Work out the finished part from the listing and answer in its coordinate system (mm). Face numbers are marked on the shaded views. Round coordinates to 2 decimals unless told otherwise and drop trailing zeros. Write each loop counter-clockwise with the first axis right and the second up, starting at its lowest first coordinate (ties: lowest second). Pieces come first, ordered by that corner, then holes.
1. Flat-ended cylindrical pins translate along their axes: pin 1 Ø7 at (x, y) = (-130, 0) entering from -Z; pin 2 Ø4 at (x, z) = (-96.5, 11.5) entering from -Y; pin 3 Ø1 at (y, z) = (64, 7) entering from -X. Find the tip coordinate at first contact, or state that the pin passes through.
2. Find section C-C (y = 0). Write down the section's boundary in (x, z).
3. Find section A-A (z = 12.5). Write down the section's boundary in (x, y).
4. Determine the mould class of the marked faces 1, 2 and 3 for opening direction Y: pulls with the +Y half, pulls with the -Y half, needs draft (parallel to the pull), parting line crosses it, or undercut.
5. Find section B-B (x = -130). Write down the section's boundary in (y, z).
6. Straight lines are drawn through the part: probe 1 along Y at (x, z) = (-130, 9.5); probe 2 along X at (y, z) = (0, 12.25); probe 3 along Z at (x, y) = (-130.5, -5). For each, find the intervals that lie inside material, in ascending order.
7. Find section D-D (y = 98). Write down the section's boundary in (x, z), and give its area (3 significant figures).
```python
from build123d import *

# Parameters (mm, degrees)
ESQUISSE2_R             = 2.75
BOSS_EXTRU_1_DEPTH      = 15
ENL_V_MAT_EXTRU_1_DEPTH = 36
CONG_1_R                = 30
CONG_2_R                = 30
CONG_3_R                = 5
CONG_4_R                = 5
CONG_5_R                = 5
CONG_6_R                = 5


with BuildPart() as part:
    # Esquisse2 → Boss.-Extru.1 (new body)
    with BuildSketch(Plane.XY):
        with BuildLine():
            Line((-125.064319956, 10), (-122, 33))
            ThreePointArc((-122, 33), (-67.197277761, 74.501212265), (0, 89))
            Line((0, 89), (0, 108))
            ThreePointArc((0, 108), (-16.165722488, 105.975834437), (-31.918403878, 101.818809198))
            ThreePointArc((-31.918403878, 101.818809198), (-87.157005326, 72.996548183), (-132.564319956, 30.332727469))
            Line((-132.564319956, 30.332727469), (-144.7, -13))
            Line((-144.7, -13), (-119, -13))
            Line((-119, -13), (-119, 4.782335439))
            Line((-119, 4.782335439), (-125.064319956, 10))
        make_face()
        with Locations((-130, 0)):
            Circle(ESQUISSE2_R, mode=Mode.SUBTRACT)
    extrude(amount=BOSS_EXTRU_1_DEPTH)

    # Esquisse5 → Enlèv. mat.-Extru.1 (cut)
    with BuildSketch(Plane(origin=(-130.800251379, 36.631666021, 0), x_dir=(0, 0, 1), z_dir=(-0.9629494993021883, 0.2696817787572327, 0))):
        Polygon((0, -51.541296877), (10, -51.541296877), (2, -6.418445839), (0, -6.541296877), align=None)
    extrude(amount=-ENL_V_MAT_EXTRU_1_DEPTH, mode=Mode.SUBTRACT)

    # Congé1
    cong_1_edges = [part.edges().sort_by_distance(p)[0] for p in [
        (-132.564319956, 30.332727469, 8.510890361),
    ]]
    fillet(cong_1_edges, radius=CONG_1_R)

    # Congé2
    cong_2_edges = [part.edges().sort_by_distance(p)[0] for p in [
        (-122, 33, 7.5),
    ]]
    fillet(cong_2_edges, radius=CONG_2_R)

    # Congé3
    cong_3_edges = [part.edges().sort_by_distance(p)[0] for p in [
        (-125.064319956, 10, 10.067243827),
    ]]
    fillet(cong_3_edges, radius=CONG_3_R)

    # Congé4
    cong_4_edges = [part.edges().sort_by_distance(p)[0] for p in [
        (-119, 4.782335439, 10.367660206),
    ]]
    fillet(cong_4_edges, radius=CONG_4_R)

    # Congé5
    cong_5_edges = [part.edges().sort_by_distance(p)[0] for p in [
        (-119, -13, 11.885604273),
    ]]
    fillet(cong_5_edges, radius=CONG_5_R)

    # Congé6
    cong_6_edges = [part.edges().sort_by_distance(p)[0] for p in [
        (-144.7, -13, 12.5),
    ]]
    fillet(cong_6_edges, radius=CONG_6_R)


solid = part.part
```
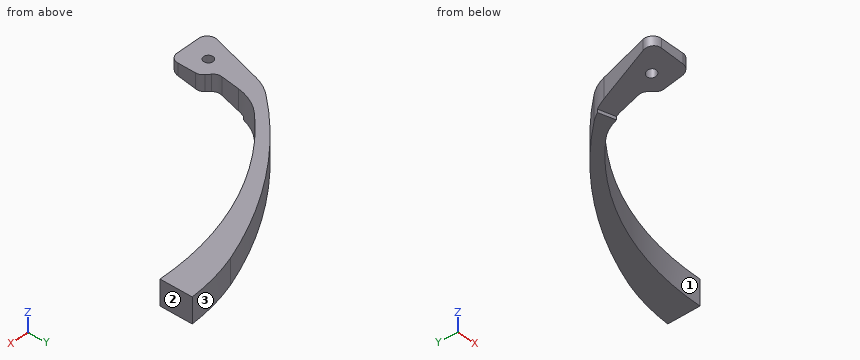
Worked answers:
1. pin 1: stops at z = 6.46
1. pin 2: stops at y = 55.49
1. pin 3: stops at x = -99.6
2. outline: (-141.06, 7.61) - (-132.75, 7.21) - (-132.75, 15) - (-141.06, 15) - close; (-127.25, 6.95) - (-119, 6.55) - (-119, 15) - (-127.25, 15) - close
3. outline: (-142.92, -6.65) arc R5 ccw to (-138.11, -13) - (-124, -13) arc R5 ccw to (-119, -8) - (-119, 2.49) arc R5 ccw to (-120.74, 6.28) - (-123.01, 8.23) arc R5 cw to (-124.71, 12.68) - (-123.23, 23.75) arc R30 cw to (-115.03, 40.67) arc R159.05 cw to (0, 89) - (0, 108) arc R122.18 ccw to (-31.92, 101.82) arc R228.65 ccw to (-128.16, 35.62) arc R30 ccw to (-134.29, 24.16) - close; hole circle Ø5.5 at (-130, 0)
4. face 1: pulls with the -Y half
4. face 2: needs draft
4. face 3: pulls with the +Y half
5. outline: (-13, 9.3) - (-2.75, 7.55) - (-2.75, 15) - (-13, 15) - close; (2.75, 6.61) - (29.74, 2) - (29.61, 0) - (33.24, 0) - (33.24, 15) - (2.75, 15) - close
6. probe 1: y = -13 to -2.75, 2.75 to 33.24
6. probe 2: x = -141.06 to -132.75, -127.25 to -119
6. probe 3: z = 7.96 to 15
7. outline: (-41.84, 0) - (0, 0) - (0, 15) - (-41.84, 15) - close
7. area: 628 mm2
